```python
from build123d import *

# Parameters (mm, degrees)
ESBO_O1_W                   = 190
ESBO_O1_H                   = 190
RESSALTO_EXTRUS_O1_DEPTH    = 5
ESBO_O2_R                   = 1
CORTE_EXTRUS_O1_DEPTH       = 276.816968296
ESBO_O3_R                   = 1
CORTE_EXTRUS_O2_DEPTH       = 5
FILETE1_R                   = 35
ESBO_O4_W                   = 19.5
ESBO_O4_H                   = 13.1
CORTE_EXTRUS_O3_DEPTH       = 276.816968296
SKETCH1_R                   = 2.35
CUT_EXTRUDE1_DEPTH          = 10
ESBO_O8_W                   = 10
ESBO_O8_H                   = 5.5
CORTE_EXTRUS_O4_DEPTH       = 276.816968296
CORTE_EXTRUS_O5_DEPTH       = 276.816968296
CORTE_EXTRUS_O7_DEPTH       = 276.816968296
CORTE_EXTRUS_O8_START       = -5
CORTE_EXTRUS_O8_OUTLINE_W   = 1.5
CORTE_EXTRUS_O8_OUTLINE_H   = 3
CORTE_EXTRUS_O8_OUTLINE_W_2 = 3
CORTE_EXTRUS_O8_OUTLINE_H_2 = 1.5
CORTE_EXTRUS_O8_DEPTH       = 5
CORTE_EXTRUS_O9_DEPTH       = 5


# Read off the part's stored shape, not the designer's step: Corte-extrusão8, Corte-extrusão9
with BuildPart() as part:
    # Esboço1 → Ressalto-extrusão1 (new body)
    with BuildSketch(Plane(origin=(0, 0, 0), x_dir=(1, 0, 0), z_dir=(0, 1, 0))):
        with Locations((100, 100)):
            Rectangle(ESBO_O1_W, ESBO_O1_H)
    extrude(amount=RESSALTO_EXTRUS_O1_DEPTH)

    # Esboço2 → Corte-extrusão1 (cut, through all)
    with BuildSketch(Plane(origin=(0, 5, 0), x_dir=(1, 0, 0), z_dir=(0, 1, 0))):
        with Locations(Location((105, 86.9, 0), (0, 0, 270))):
            Circle(ESBO_O2_R)
        with Locations(Location((105, 134.3, 0), (0, 0, 270))):
            Circle(ESBO_O2_R)
        with Locations(Location((95, 86.9, 0), (0, 0, 90))):
            Circle(ESBO_O2_R)
        with Locations(Location((95, 134.3, 0), (0, 0, 90))):
            Circle(ESBO_O2_R)
        with BuildLine():
            Line((90, 131.1), (110, 131.1))
            Line((110, 131.1), (110, 90.1))
            Line((110, 90.1), (104, 90.1))
            ThreePointArc((104, 90.1), (103.292893219, 89.807106781), (103, 89.1))
            Line((103, 89.1), (103, 88.6))
            ThreePointArc((103, 88.6), (102.326345597, 86.973654403), (100.7, 86.3))
            Line((100.7, 86.3), (99.3, 86.3))
            ThreePointArc((99.3, 86.3), (97.673654403, 86.973654403), (97, 88.6))
            Line((97, 88.6), (97, 89.1))
            ThreePointArc((97, 89.1), (96.707106781, 89.807106781), (96, 90.1))
            Line((96, 90.1), (90, 90.1))
            Line((90, 90.1), (90, 131.1))
        make_face()
    extrude(amount=-CORTE_EXTRUS_O1_DEPTH, mode=Mode.SUBTRACT)

    # Esboço3 → Corte-extrusão2 (cut)
    with BuildSketch(Plane(origin=(0, 5, 0), x_dir=(1, 0, 0), z_dir=(0, 1, 0))):
        with Locations(Location((45, 182.5, 0), (0, 0, 270))):
            Circle(ESBO_O3_R)
        with Locations(Location((45, 17.5, 0), (0, 0, 90))):
            Circle(ESBO_O3_R)
        with Locations(Location((155, 17.5, 0), (0, 0, 270))):
            Circle(ESBO_O3_R)
        with Locations(Location((155, 182.5, 0), (0, 0, 90))):
            Circle(ESBO_O3_R)
    extrude(amount=-CORTE_EXTRUS_O2_DEPTH, mode=Mode.SUBTRACT)

    # Filete1
    filete1_edges = [part.edges().sort_by_distance(p)[0] for p in [
        (5, 2.5, -195),
        (195, 2.5, -195),
        (195, 2.5, -5),
        (5, 2.5, -5),
    ]]
    fillet(filete1_edges, radius=FILETE1_R)

    # Esboço4 → Corte-extrusão3 (cut, through all)
    with BuildSketch(Plane(origin=(0, 5, 0), x_dir=(1, 0, 0), z_dir=(0, 1, 0))):
        with Locations((130, 182.5)):
            Rectangle(ESBO_O4_W, ESBO_O4_H)
    extrude(amount=-CORTE_EXTRUS_O3_DEPTH, mode=Mode.SUBTRACT)

    # Sketch1 → Cut-Extrude1 (cut)
    with BuildSketch(Plane(origin=(0, 5, 0), x_dir=(1, 0, 0), z_dir=(0, 1, 0))):
        with Locations(Location((110.25, 177.79006803, 0), (0, 0, 90))):
            Circle(SKETCH1_R)
        with Locations(Location((57.782465694, 186.314872597, 0), (0, 0, 270))):
            Circle(SKETCH1_R)
        with Locations(Location((110.25, 186.314872597, 0), (0, 0, 270))):
            Circle(SKETCH1_R)
    extrude(amount=-CUT_EXTRUDE1_DEPTH, mode=Mode.SUBTRACT)

    # Esboço8 → Corte-extrusão4 (cut, through all)
    with BuildSketch(Plane(origin=(0, 5, 0), x_dir=(-1, 0, 0), z_dir=(0, 1, 0))):
        with Locations((-67.499895869, -164.49975707)):
            Rectangle(ESBO_O8_W, ESBO_O8_H)
        with Locations((-67.499895869, -74.50024293)):
            Rectangle(ESBO_O8_W, ESBO_O8_H)
    extrude(amount=-CORTE_EXTRUS_O4_DEPTH, mode=Mode.SUBTRACT)

    # Esboço10 → Corte-extrusão5 (cut, through all)
    with BuildSketch(Plane(origin=(0, 5, 0), x_dir=(1, 0, 0), z_dir=(0, 1, 0))):
        with BuildLine():
            Line((29.81236761, 53.368860086), (39.621292879, 57.27884335))
            ThreePointArc((39.621292879, 57.27884335), (40.643023517, 59.216773827), (38.64138653, 60.107255383))
            Line((38.64138653, 60.107255383), (31.023574835, 56.885452176))
            ThreePointArc((31.023574835, 56.885452176), (30.081566568, 56.972943613), (29.634049405, 57.806467887))
            Line((29.634049405, 57.806467887), (29.634049405, 67.297779802))
            ThreePointArc((29.634049405, 67.297779802), (29.341156187, 68.004886583), (28.634049405, 68.297779802))
            Line((28.634049405, 68.297779802), (20.634049405, 68.297779802))
            ThreePointArc((20.634049405, 68.297779802), (19.926942624, 68.004886583), (19.634049405, 67.297779802))
            Line((19.634049405, 67.297779802), (19.634049405, 54.297779802))
            ThreePointArc((19.634049405, 54.297779802), (19.926942624, 53.590673021), (20.634049405, 53.297779802))
            Line((20.634049405, 53.297779802), (29.442086417, 53.297779802))
            ThreePointArc((29.442086417, 53.297779802), (29.63060735, 53.31571063), (29.81236761, 53.368860086))
        make_face()
    extrude(amount=-CORTE_EXTRUS_O5_DEPTH, mode=Mode.SUBTRACT)

    # Esboço12 → Corte-extrusão7 (cut, through all)
    with BuildSketch(Plane(origin=(0, 5, 0), x_dir=(1, 0, 0), z_dir=(0, 1, 0))):
        with BuildLine():
            Line((115, 123.1), (115, 98.1))
            ThreePointArc((115, 98.1), (120, 93.1), (125, 98.1))
            Line((125, 98.1), (125, 123.1))
            ThreePointArc((125, 123.1), (120, 128.1), (115, 123.1))
        make_face()
    extrude(amount=-CORTE_EXTRUS_O7_DEPTH, mode=Mode.SUBTRACT)

    # Corte-extrusão8 outline → Corte-extrusão8 (cut)
    with BuildSketch(Plane(origin=(0, 5, 0), x_dir=(1, 0, 0), z_dir=(0, 1, 0)).offset(CORTE_EXTRUS_O8_START)):
        Polygon((93.630915931, 184.471333361), (93.557673586, 182.973122575), (96.554095158, 182.826637886), (96.627337502, 184.324848672), align=None)
        Polygon((96.309954009, 177.832601933), (93.313532437, 177.979086622), (93.240290093, 176.480875836), (96.236711664, 176.334391147), align=None)
        with Locations((114.04726065, 157.727587795)):
            Rectangle(CORTE_EXTRUS_O8_OUTLINE_W, CORTE_EXTRUS_O8_OUTLINE_H)
        with Locations((107.54726065, 157.727587795)):
            Rectangle(CORTE_EXTRUS_O8_OUTLINE_W, CORTE_EXTRUS_O8_OUTLINE_H)
        with Locations((100.460308888, 62.543165179)):
            Rectangle(CORTE_EXTRUS_O8_OUTLINE_W_2, CORTE_EXTRUS_O8_OUTLINE_H_2)
        with Locations((73.101842496, 62.543165179)):
            Rectangle(CORTE_EXTRUS_O8_OUTLINE_W_2, CORTE_EXTRUS_O8_OUTLINE_H_2)
        with Locations((100.460308888, 56.043165179)):
            Rectangle(CORTE_EXTRUS_O8_OUTLINE_W_2, CORTE_EXTRUS_O8_OUTLINE_H_2)
        with Locations((73.101842496, 56.043165179)):
            Rectangle(CORTE_EXTRUS_O8_OUTLINE_W_2, CORTE_EXTRUS_O8_OUTLINE_H_2)
        with Locations((142, 51.488873394)):
            Rectangle(CORTE_EXTRUS_O8_OUTLINE_W_2, CORTE_EXTRUS_O8_OUTLINE_H_2)
        with Locations((142, 44.988873394)):
            Rectangle(CORTE_EXTRUS_O8_OUTLINE_W_2, CORTE_EXTRUS_O8_OUTLINE_H_2)
    extrude(amount=CORTE_EXTRUS_O8_DEPTH, mode=Mode.SUBTRACT)

    # Corte-extrusão9 outline → Corte-extrusão9 (cut)
    with BuildSketch(Plane(origin=(0, 0, 0), x_dir=(1, 0, 0), z_dir=(0, 1, 0))):
        with BuildLine():
            Line((102.439246138, 71.3), (118.732019964, 71.3))
            ThreePointArc((118.732019964, 71.3), (123.732019964, 76.3), (118.732019964, 81.3))
            Line((118.732019964, 81.3), (102.439246138, 81.3))
            ThreePointArc((102.439246138, 81.3), (97.439246138, 76.3), (102.439246138, 71.3))
        make_face()
    extrude(amount=CORTE_EXTRUS_O9_DEPTH, mode=Mode.SUBTRACT)


solid = part.part
```
Geometry check sheet. Reference: the model listing, model coordinates, mm. A direction names the side the tool comes from. Give positions to 0.01 mm unless a question says otherwise; leave off trailing zeros. Order: outer loops, then holes, each group sorted by start corner. A loop starts at its lowest first (then second) coordinate and runs counter-clockwise, first axis right, second up. Notation, with made-up numbers: (37, 15.5) - (42, 15.5) arc R13 ccw to (42, 32.5) - close; hole circle Ø5 at (85.5, 35). An arc over 180 degrees is marked (long way). Answer in a Markdown table with one row per item. Add a question column.
Q1. Mould release check, pull along X, two halves, no side actions. Record for faces 1 (the flat face through (25, 3, -53.298)), 2 (the flat face through (98.7, 0, -80.2)): pulls with the +X half, pulls with the -X half, needs draft (parallel to the pull), parting line crosses it, or undercut.
Q2. Gauge pin test, flat ends, axial feed: pin 1 (5.5 mm diameter, centred on x = 57.78, z = -186.31, fed in from +Y); pin 2 (1.5 mm diameter, centred on y = 3, z = -165, fed in from +X). Record the tip position at first contact, or that the pin passes through.
Q3. Cross-section at B-B, the plane y = 1.8. Count the separate pieces of the cut face and the enclosed holes in it, then the cut area to 3 significant figures.
Q4. Material ranges on probe 1 along Z at (x, y) = (105, 2.5); probe 2 along X at (y, z) = (4.25, -76); probe 3 along X at (y, z) = (4.35, -58.5), recorded low to high. Write a range as from..to.
Q5. Tool access check on faces 3 (the flat face through (99, 2, -5)), 4 (the flat face through (29.634, 3, -62)). Record the directions out of +Z, -Z, +X, -X, +Y, -Y that give a thin tool (end or side, any length) a straight path to the whole face; none if there is none.
Q6. Cross-section at A-A, the plane z = -116.5. Enter the section's corners in (x, y), then the cut area to 3 significant figures.
Check values:
| question | item | result |
|---|---|---|
| 1 | face 1 | undercut |
| 1 | face 2 | needs draft |
| 2 | pin 1 | stops at y = 5 |
| 2 | pin 2 | stops at x = 194.74 |
| 3 | separate pieces | 1 |
| 3 | enclosed holes | 28 |
| 3 | area | 33,000 mm^2 |
| 4 | probe 1 | z = -195..-135.3, -133.3..-131.1, -90.1..-87.9, -85.9..-81.3, -71.3..-5 |
| 4 | probe 2 | x = 5..62.5, 72.5..97.45, 123.72..195 |
| 4 | probe 3 | x = 5..19.63, 29.63..34.84, 40.71..195 |
| 5 | face 3 | +Z, +X, -X, +Y, -Y |
| 5 | face 4 | +Y, -Y |
| 6 | outline | (5, 0) - (90, 0) - (90, 5) - (5, 5) - close; (110, 0) - (115, 0) - (115, 5) - (110, 5) - close; (125, 0) - (195, 0) - (195, 5) - (125, 5) - close |
| 6 | area | 800 mm^2 |
